Check sheet for the drawn part. Datum: minimum x, y, z corner. Units: mm. Give positions to 0.01 mm unless a question says otherwise; leave off trailing zeros. Loops run counter-clockwise (first coordinate to the right, second up) from the corner with the lowest first, then second, coordinate; pieces in that order, holes last. Notation, with made-up numbers: (72, -24) - (116, -24) arc R27 cw to (116, -7) - close; hole circle Ø10 at (10, 56). An arc over 180 degrees is marked (long way). Answer in a Markdown table with one row per item.
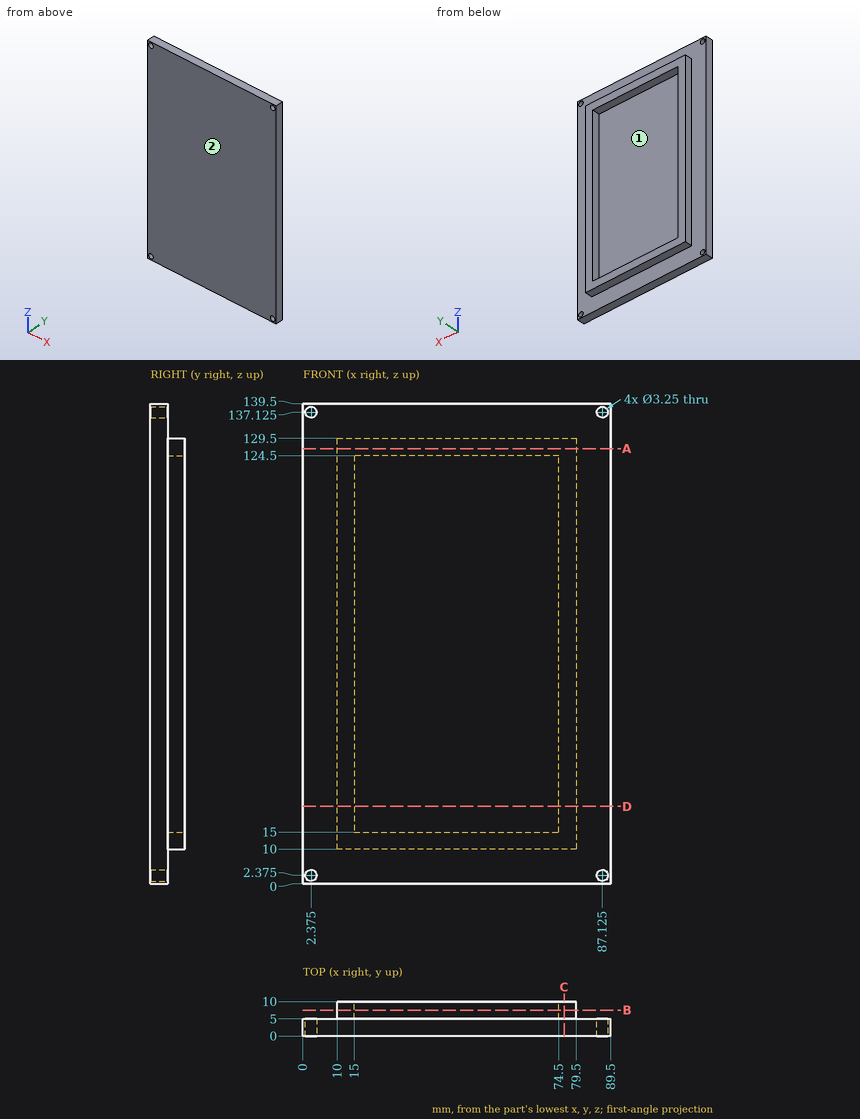
Q1. Go/stop test with flat-tipped pins: P1, Ø5.5, axis at y = 8, z = 55.5, coming from the -X side; P2, Ø4, axis at y = 8.5, z = 75.5, coming from the +X side; P3, Ø2.5, axis at x = 34.5, y = 8, coming from the -Z side. Record where each tip stops, or that it passes through.
Completed:
| item | result |
|---|---|
| P1 | x = 10 |
| P2 | x = 79.5 |
| P3 | z = 10 |
Q2. Thickness scan on line 1 (X direction, y = 6, z = 109); line 2 (Z direction, x = 32, y = 9.25); line 3 (Y direction, x = 33.5, z = 102). Record the ranges inside material, lowest first.
Completed:
| item | result |
|---|---|
| line 1 | 10 to 15, 74.5 to 79.5 |
| line 2 | 10 to 15, 124.5 to 129.5 |
| line 3 | 0 to 5 |
Q3. Sectioned sample at B-B (y = 7.5). Record the cut outline in (x, z).
Completed:
| item | result |
|---|---|
| outline | (10, 10) - (79.5, 10) - (79.5, 129.5) - (10, 129.5) - close; hole (15, 15) - (74.5, 15) - (74.5, 124.5) - (15, 124.5) - close |
Q4. Sectioned sample at A-A (z = 126.5). Record the cut outline in (x, y).
Completed:
| item | result |
|---|---|
| outline | (0, 0) - (89.5, 0) - (89.5, 5) - (79.5, 5) - (79.5, 10) - (10, 10) - (10, 5) - (0, 5) - close |
Q5. Sectioned sample at D-D (z = 22.5). Record the cut outline in (x, y).
Completed:
| item | result |
|---|---|
| outline | (0, 0) - (89.5, 0) - (89.5, 5) - (79.5, 5) - (79.5, 10) - (74.5, 10) - (74.5, 5) - (15, 5) - (15, 10) - (10, 10) - (10, 5) - (0, 5) - close |
Q6. Sectioned sample at C-C (x = 76). Record the cut outline in (y, z).
Completed:
| item | result |
|---|---|
| outline | (0, 0) - (5, 0) - (5, 10) - (10, 10) - (10, 129.5) - (5, 129.5) - (5, 139.5) - (0, 139.5) - close |
Q7. Draft check along Z on the marked faces 1 and 2. Enter one of: +Z half, -Z half, draft (parallel to the pull), parting line (faces both ways), or undercut.
Completed:
| item | result |
|---|---|
| face 1 | undercut |
| face 2 | draft |
